```python
from build123d import *

# Parameters (mm, degrees)
SKETCH1_R           = 18
BOSS_EXTRUDE1_DEPTH = 3
CUT_EXTRUDE1_START  = -3
CUT_EXTRUDE1_DEPTH  = 3
CIRPATTERN1_COUNT   = 10
CUT_EXTRUDE3_DEPTH  = 26.171545449


with BuildPart() as part:
    # Sketch1 → Boss-Extrude1 (new body)
    with BuildSketch(Plane.XY):
        Circle(SKETCH1_R)
    extrude(amount=BOSS_EXTRUDE1_DEPTH)

    # Sketch2 → Cut-Extrude1 (cut)
    with BuildSketch(Plane.XY.offset(3).offset(CUT_EXTRUDE1_START)):
        with BuildLine():
            ThreePointArc((4.836662041, 17.338013159), (2.183107171, 14.775836074), (1.52990268, 11.145487777))
            ThreePointArc((1.52990268, 11.145487777), (0, 11.25), (-1.52990268, 11.145487777))
            ThreePointArc((-1.52990268, 11.145487777), (-2.183107171, 14.775836074), (-4.836662041, 17.338013159))
            ThreePointArc((-4.836662041, 17.338013159), (0, 18), (4.836662041, 17.338013159))
        make_face()
    cut_extrude1 = extrude(amount=CUT_EXTRUDE1_DEPTH, mode=Mode.SUBTRACT)

    # CirPattern1: Cut-Extrude1 ×10 about axis
    cirpattern1_axis = Axis((0, 0, 0), (0, 0, 1))
    for i in range(1, CIRPATTERN1_COUNT):
        add(cut_extrude1.rotate(cirpattern1_axis, i * 360 / CIRPATTERN1_COUNT), mode=Mode.SUBTRACT)

    # Sketch4 → Cut-Extrude3 (cut, through all)
    with BuildSketch(Plane.XY.offset(3)):
        with BuildLine():
            Line((-0.241039416, 2.9), (0.241039416, 2.9))
            ThreePointArc((0.241039416, 2.9), (0, -2.91), (-0.241039416, 2.9))
        make_face()
    extrude(amount=-CUT_EXTRUDE3_DEPTH, mode=Mode.SUBTRACT)


solid = part.part
```
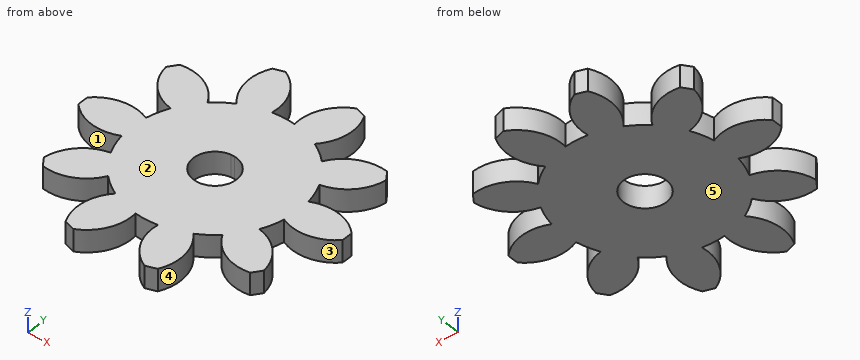
Here's how the part is built. I have some questions about the finished solid (model axes, mm). Face numbers are marked on the shaded views. A direction names the side the tool comes from. Coordinates: 2 decimals unless noted, no trailing zeros. Loops run counter-clockwise (first coordinate to the right, second up) from the corner with the lowest first, then second, coordinate; pieces in that order, holes last. Notation, with made-up numbers: (22, 59) -> (72, 59) arc R6 ccw to (72, 67) -> close; hole circle Ø9 at (77.5, 8.5). An arc over 180 degrees is marked (long way). Return JSON: item names as keys, results as strings.
1) If we section it at D-D, the plane x = 4: Write out the boundary of the cut face in (y, z), then the cut area to 3 significant figures.
Results below:
{"outline": "(-16.84, 0) -> (16.84, 0) -> (16.84, 3) -> (-16.84, 3) -> close", "area": "101 mm²"}
2) If we section it at B-B, the plane y = -9: Write out the boundary of the cut face in (x, z).
Results below:
{"outline": "(-14.78, 0) -> (-8.37, 0) -> (-8.37, 3) -> (-14.78, 3) -> close; (-6.75, 0) -> (6.75, 0) -> (6.75, 3) -> (-6.75, 3) -> close; (8.37, 0) -> (14.78, 0) -> (14.78, 3) -> (8.37, 3) -> close"}
3) If we section it at A-A, the plane y = 0: Write out the boundary of the cut face in (x, z).
Results below:
{"outline": "(-18, 0) -> (-2.91, 0) -> (-2.91, 3) -> (-18, 3) -> close; (2.91, 0) -> (18, 0) -> (18, 3) -> (2.91, 3) -> close"}
4) Thinking about a two-plate mould opening in Y: for the marked faces 1, 2 and 3, which applies, +Y half, -Y half, draft (parallel to the pull), parting line (faces both ways), or undercut?
Results below:
{"face 1": "undercut", "face 2": "draft", "face 3": "undercut"}
5) Will these pins go through, and if not, where does the flat tip stop? pin 1 (1 mm diameter, centred on y = -5, z = 1, fed in from -X); pin 2 (1 mm diameter, centred on x = -5.5, z = 2, fed in from -Y).
Results below:
{"pin 1": "x = -11.86", "pin 2": "y = -17.29"}
6) I need wall thicknesses on line 1 (Y direction, x = 0, z = 1.5); line 2 (X direction, y = 0, z = 1.8); line 3 (Y direction, x = -14.5, z = 1.75). Which ranges of each line are inside material? Lowest first, please. Write a range as from..to.
Results below:
{"line 1": "-11.25..-2.91, 2.9..11.25", "line 2": "-18..-2.91, 2.91..18", "line 3": "-10.67..-8.28, -2.53..2.53, 8.28..10.67"}
7) For the marked faces 4 and 5, which set-ups out of +Z, -Z, +X, -X, +Y, -Y let a thin tool reach every point of the face, with its end or its side?
Results below:
{"face 4": "+Z, -Z", "face 5": "-Z, +X, -X, +Y, -Y"}
8) If we section it at C-C, the plane y = 15: Write out the boundary of the cut face in (x, z), then the cut area to 3 significant figures.
Results below:
{"outline": "(-6.9, 0) -> (-2.31, 0) -> (-2.31, 3) -> (-6.9, 3) -> close; (2.31, 0) -> (6.9, 0) -> (6.9, 3) -> (2.31, 3) -> close", "area": "27.6 mm²"}
